```python
from build123d import *

# Parameters (mm, degrees)
ESQUISSE1_R             = 1.5
ESQUISSE1_R_2           = 1.50110642
BOSS_EXTRU_1_DEPTH      = 4
ENL_V_MAT_EXTRU_1_REACH = 124.989
ESQUISSE2_R             = 1.5


with BuildPart() as part:
    # Esquisse1 → Boss.-Extru.1 (new body)
    with BuildSketch(Plane.XY):
        with BuildLine():
            ThreePointArc((60.026944648, 49.921558504), (72.778337749, 29.898863696), (84.195273994, 9.086369847))
            ThreePointArc((84.195273994, 9.086369847), (91.451273571, 4.140927091), (99.509067829, 7.630753106))
            ThreePointArc((99.509067829, 7.630753106), (105.251720368, 19.156706799), (106.145904128, 32.002955361))
            ThreePointArc((106.145904128, 32.002955361), (105.517176975, 33.787686969), (104.210334733, 35.15616353))
            ThreePointArc((104.210334733, 35.15616353), (92.58899703, 44.531440422), (81.889188019, 54.946112475))
            ThreePointArc((81.889188019, 54.946112475), (80.829609942, 55.239205413), (80.085451585, 54.429985101))
            ThreePointArc((80.085451585, 54.429985101), (79.43974416, 52.594599516), (78.30149473, 51.016636729))
            ThreePointArc((78.30149473, 51.016636729), (76.19777745, 50.272546762), (74.337717048, 51.505215238))
            ThreePointArc((74.337717048, 51.505215238), (73.781586954, 52.671085372), (73.412965229, 53.909088553))
            ThreePointArc((73.412965229, 53.909088553), (71.258227235, 58.277263879), (67.291581582, 61.103847288))
            ThreePointArc((67.291581582, 61.103847288), (62.173852637, 60.880940246), (58.891944342, 56.947758957))
            ThreePointArc((58.891944342, 56.947758957), (58.674610839, 53.307878055), (60.026944648, 49.921558504))
        make_face()
        with Locations((68.285467108, 55.560427953)):
            Circle(ESQUISSE1_R, mode=Mode.SUBTRACT)
        with Locations((101.682075096, 31.433543054)):
            Circle(ESQUISSE1_R, mode=Mode.SUBTRACT)
        with Locations((92.312371453, 13.200094295)):
            Circle(ESQUISSE1_R, mode=Mode.SUBTRACT)
        with Locations((67.535467108, 46.360427953)):
            Circle(ESQUISSE1_R_2, mode=Mode.SUBTRACT)
        with BuildLine():
            Line((96.849719723, 30.848999233), (96.849719723, 33.474650871))
            ThreePointArc((96.849719723, 33.474650871), (96.647309876, 34.343108764), (96.081794601, 35.032587793))
            ThreePointArc((96.081794601, 35.032587793), (89.436975045, 40.671042336), (83.372922141, 46.929880801))
            ThreePointArc((83.372922141, 46.929880801), (81.323140328, 47.752609653), (79.445810973, 46.588941858))
            ThreePointArc((79.445810973, 46.588941858), (77.571604785, 42.607109512), (76.591708968, 38.316720036))
            ThreePointArc((76.591708968, 38.316720036), (76.69683067, 36.288635677), (77.467153905, 34.409598995))
            ThreePointArc((77.467153905, 34.409598995), (79.992055499, 30.078906011), (82.254048976, 25.605270433))
            ThreePointArc((82.254048976, 25.605270433), (84.350090923, 23.753861276), (87.134236378, 24.017758597))
            ThreePointArc((87.134236378, 24.017758597), (91.023623533, 25.188476532), (95.051173024, 24.662398573))
            ThreePointArc((95.051173024, 24.662398573), (97.816197879, 25.543673578), (97.709238653, 28.443771474))
            ThreePointArc((97.709238653, 28.443771474), (97.07105369, 29.571903567), (96.849719723, 30.848999233))
        make_face(mode=Mode.SUBTRACT)
    extrude(amount=BOSS_EXTRU_1_DEPTH)

    # Esquisse2 → Enlèv. mat.-Extru.1 (cut, up to next)
    with BuildSketch(Plane.XY.offset(4), mode=Mode.PRIVATE) as enl_v_mat_extru_1_sk1:
        with Locations((76.312371453, 30.200094295)):
            Circle(ESQUISSE2_R)
    enl_v_mat_extru_1_tool1 = extrude(enl_v_mat_extru_1_sk1.sketch, amount=-ENL_V_MAT_EXTRU_1_REACH, mode=Mode.PRIVATE) & part.part
    add(enl_v_mat_extru_1_tool1.solids().sort_by_distance((76.312371, 30.200094, 4))[0], mode=Mode.SUBTRACT)


solid = part.part
```
Verification items for the finished model (mm, model axes). A direction names the side the tool comes from. Coordinates: 2 decimals unless noted, no trailing zeros. Order: outer loops, then holes, each group sorted by start corner. A loop starts at its lowest first (then second) coordinate and runs counter-clockwise, first axis right, second up. Notation, with made-up numbers: (-25, 89.5) - (-13, 89.5) arc R15 cw to (-13, 111.5) - close; hole circle Ø7 at (87.25, 0). An arc over 180 degrees is marked (long way). Return JSON: item names as keys, results as strings.
(1) Thickness scan on line 1 along X through (y, z) = (47, 1.2); line 2 along Y through (x, z) = (82, 0.45); line 3 along X through (y, z) = (34, 3.05). Record the ranges inside material, lowest first.
Filled sheet:
{"line 1": "x = 62 to 66.18, 68.89 to 79.76, 83.31 to 89.87", "line 2": "y = 13.35 to 26.14, 47.72 to 54.83", "line 3": "x = 70.31 to 77.72, 96.78 to 105.38"}
(2) Go/stop test with flat-tipped pins: pin 1 (1 mm diameter, centred on x = 96.5, z = 3.5, fed in from -Y); pin 2 (2.5 mm diameter, centred on x = 101.68, y = 31.43, fed in from +Z); pin 3 (2 mm diameter, centred on y = 32.5, z = 3, fed in from -X). Record where each tip stops, or that it passes through.
Filled sheet:
{"pin 1": "stops at y = 4.88", "pin 2": "passes through", "pin 3": "stops at x = 70.62"}
(3) Section check D-D, the plane x = 63. Record the cut outline in (y, z), and give its area (3 significant figures).
Filled sheet:
{"outline": "(45.5, 0) - (61.22, 0) - (61.22, 4) - (45.5, 4) - close", "area": "62.9 mm^2"}
(4) Section check C-C, the plane z = 2.9. Record the cut outline in (x, y).
Filled sheet:
{"outline": "(58.89, 56.95) arc R8.36 ccw to (60.03, 49.92) arc R363.4 cw to (84.2, 9.09) arc R9.1 ccw to (99.51, 7.63) arc R33 ccw to (106.15, 32) arc R4.5 ccw to (104.21, 35.16) arc R160.5 cw to (81.89, 54.95) arc R1.05 ccw to (80.09, 54.43) arc R6.81 cw to (78.3, 51.02) arc R2.5 cw to (74.34, 51.51) arc R8.31 cw to (73.41, 53.91) arc R9.97 ccw to (67.29, 61.1) arc R6.34 ccw to start; hole circle Ø3 at (67.54, 46.36); hole circle Ø3 at (68.29, 55.56); hole circle Ø3 at (76.31, 30.2); hole (76.59, 38.32) arc R6.05 ccw to (77.47, 34.41) arc R83.98 cw to (82.25, 25.61) arc R3.52 ccw to (87.13, 24.02) arc R9.69 cw to (95.05, 24.66) arc R2.4 ccw to (97.71, 28.44) arc R3.8 cw to (96.85, 30.85) - (96.85, 33.47) arc R1.96 ccw to (96.08, 35.03) arc R89.37 cw to (83.37, 46.93) arc R2.45 ccw to (79.45, 46.59) arc R20.47 ccw to start; hole circle Ø3 at (92.31, 13.2); hole circle Ø3 at (101.68, 31.43)"}
(5) Mould release check, pull along X, two halves, no side actions. Record for faces 4 (the cylindrical face through (80.845, 55.244, 1.972)), 5 (the cylindrical face through (84.312, 23.767, 1.972)), 6 (the cylindrical face through (62.24, 60.913, 1.972)), 7 (the cylindrical face through (58.667, 53.359, 1.972)): pulls with the +X half, pulls with the -X half, needs draft (parallel to the pull), parting line crosses it, or undercut.
Filled sheet:
{"face 4": "undercut", "face 5": "undercut", "face 6": "parting line crosses it", "face 7": "pulls with the -X half"}
(6) Section check B-B, the plane x = 75.5. Record the cut outline in (y, z), and give its area (3 significant figures).
Filled sheet:
{"outline": "(25.22, 0) - (28.94, 0) - (28.94, 4) - (25.22, 4) - close; (31.46, 0) - (50.46, 0) - (50.46, 4) - (31.46, 4) - close", "area": "90.9 mm^2"}
(7) Section check A-A, the plane y = 45.5. Record the cut outline in (x, z), and give its area (3 significant figures).
Filled sheet:
{"outline": "(63, 0) - (66.31, 0) - (66.31, 4) - (63, 4) - close; (68.77, 0) - (78.83, 0) - (78.83, 4) - (68.77, 4) - close; (84.66, 0) - (91.51, 0) - (91.51, 4) - (84.66, 4) - close", "area": "80.9 mm^2"}
(8) Access from +Z, -Z, +X, -X, +Y, -Y to the whole of each face (thin tool, end or side, straight path). Record for faces 1 (the cylindrical face through (79.96, 30.14, 1.97)), 2 (the cylindrical face through (91.324, 4.154, 1.972)), 3 (the cylindrical face through (79.452, 52.619, 1.972)).
Filled sheet:
{"face 1": "+Z, -Z", "face 2": "+Z, -Z, -Y", "face 3": "+Z, -Z, +Y"}
